Part model, mm, in its own coordinate system. Give positions to 0.01 mm unless a question says otherwise; leave off trailing zeros. Loops run counter-clockwise (first coordinate to the right, second up) from the corner with the lowest first, then second, coordinate; pieces in that order, holes last. Notation, with made-up numbers: (-5.5, -21) -> (7.5, -21) arc R11 cw to (7.5, -4) -> close; hole circle Ø5 at (28, 44.5). An arc over 180 degrees is marked (long way). One line per question, with ' | ' between items.
```python
from build123d import *

# Parameters (mm, degrees)
SKETCH_1_R          = 1.5
SKETCH_1_R_2        = 1
EXTRUDE_1_DEPTH     = 3
SKETCH_2_R          = 1.5
CUT_EXTRUDE_2_DEPTH = 10
SKETCH_2_6_R        = 2.5
CUT_EXTRUDE_3_DEPTH = 10
SKETCH_2_7_R        = 2.5
CUT_EXTRUDE_4_DEPTH = 10


with BuildPart() as part:
    # Sketch 1 → Extrude 1 (new body)
    with BuildSketch(Plane.XY):
        with BuildLine():
            Line((-102, -62), (-8, -62))
            ThreePointArc((-8, -62), (-5.878679656, -61.121320344), (-5, -59))
            Line((-5, -59), (-5, 85))
            ThreePointArc((-5, 85), (-5.878679656, 87.121320344), (-8, 88))
            Line((-8, 88), (-102, 88))
            ThreePointArc((-102, 88), (-104.121320344, 87.121320344), (-105, 85))
            Line((-105, 85), (-105, -59))
            ThreePointArc((-105, -59), (-104.121320344, -61.121320344), (-102, -62))
        make_face()
        with Locations(Location((-100.157022476, 13, 0), (0, 0, 180))):
            Circle(SKETCH_1_R, mode=Mode.SUBTRACT)
        with Locations(Location((-12, 81, 0), (0, 0, 180))):
            Circle(SKETCH_1_R, mode=Mode.SUBTRACT)
        with Locations(Location((-98, -55, 0), (0, 0, 180))):
            Circle(SKETCH_1_R, mode=Mode.SUBTRACT)
        with Locations(Location((-98, 81, 0), (0, 0, 180))):
            Circle(SKETCH_1_R, mode=Mode.SUBTRACT)
        with Locations(Location((-12, -55, 0), (0, 0, 180))):
            Circle(SKETCH_1_R, mode=Mode.SUBTRACT)
        with Locations(Location((-10, 6, 0), (0, 0, 180))):
            Circle(SKETCH_1_R_2, mode=Mode.SUBTRACT)
        with Locations(Location((-20, 20, 0), (0, 0, 180))):
            Circle(SKETCH_1_R_2, mode=Mode.SUBTRACT)
        with Locations(Location((-20, 6, 0), (0, 0, 180))):
            Circle(SKETCH_1_R_2, mode=Mode.SUBTRACT)
        with Locations(Location((-10, 20, 0), (0, 0, 180))):
            Circle(SKETCH_1_R_2, mode=Mode.SUBTRACT)
    extrude(amount=-EXTRUDE_1_DEPTH)

    # Sketch 2 → Cut-Extrude 2 (cut)
    with BuildSketch(Plane.XY):
        with Locations((-90.41, 69.42)):
            Circle(SKETCH_2_R)
        with Locations((-18.41, 69.42)):
            Circle(SKETCH_2_R)
        with Locations((-90.41, -44.58)):
            Circle(SKETCH_2_R)
        with Locations((-18.41, -44.58)):
            Circle(SKETCH_2_R)
    extrude(amount=-CUT_EXTRUDE_2_DEPTH, mode=Mode.SUBTRACT)

    # Sketch 2_6 → Cut-Extrude 3 (cut)
    with BuildSketch(Plane.XY):
        with Locations((-83.178616271, -57.326639146)):
            Circle(SKETCH_2_6_R)
        with Locations((-26.33472009, -57.326639146)):
            Circle(SKETCH_2_6_R)
    extrude(amount=-CUT_EXTRUDE_3_DEPTH, mode=Mode.SUBTRACT)

    # Sketch 2_7 → Cut-Extrude 4 (cut)
    with BuildSketch(Plane.XY):
        with Locations((-83.178616271, 83.33)):
            Circle(SKETCH_2_7_R)
        with Locations((-26.33472009, 83.33)):
            Circle(SKETCH_2_7_R)
    extrude(amount=-CUT_EXTRUDE_4_DEPTH, mode=Mode.SUBTRACT)


solid = part.part
```
1) Pull direction Y, two halves, no side cores. Call faces 1 (the flat face through (-54, 88, -1)), 2 (the cylindrical face through (-19.6, -45.49, -1.48)), 3 (the cylindrical face through (-5.9, -61.14, -1.48)): pulls with the +Y half, pulls with the -Y half, needs draft (parallel to the pull), parting line crosses it, or undercut.
Found:
face 1: pulls with the +Y half | face 2: undercut | face 3: pulls with the -Y half
2) Saw through at B-B (y = 13). Give the cut face in (x, z), and give its area (3 significant figures).
Found:
outline: (-105, -3) -> (-101.66, -3) -> (-101.66, 0) -> (-105, 0) -> close; (-98.66, -3) -> (-5, -3) -> (-5, 0) -> (-98.66, 0) -> close | area: 291 mm2
3) Drill centre lines: line 1 (X direction, y = 69.42, z = -0.7); line 2 (Y direction, x = -10, z = -1.7); line 3 (Y direction, x = -12, z = -1.75). Where is each one in solid material? Low to high.
Found:
line 1: -105 to -91.91, -88.91 to -19.91, -16.91 to -5 | line 2: -62 to 5, 7 to 19, 21 to 88 | line 3: -62 to -56.5, -53.5 to 79.5, 82.5 to 88
4) Saw through at C-C (x = -84). Give the cut face in (y, z), and give its area (3 significant figures).
Found:
outline: (-62, -3) -> (-59.69, -3) -> (-59.69, 0) -> (-62, 0) -> close; (-54.97, -3) -> (80.97, -3) -> (80.97, 0) -> (-54.97, 0) -> close; (85.69, -3) -> (88, -3) -> (88, 0) -> (85.69, 0) -> close | area: 422 mm2
5) Saw through at A-A (y = 69.42). Give the cut face in (x, z), and give its area (3 significant figures).
Found:
outline: (-105, -3) -> (-91.91, -3) -> (-91.91, 0) -> (-105, 0) -> close; (-88.91, -3) -> (-19.91, -3) -> (-19.91, 0) -> (-88.91, 0) -> close; (-16.91, -3) -> (-5, -3) -> (-5, 0) -> (-16.91, 0) -> close | area: 282 mm2
